For this review, take the finished solid that the model builds, in its own axes (mm). A direction names the side the tool comes from. Round coordinates to 2 decimals unless told otherwise and drop trailing zeros. Write each loop counter-clockwise with the first axis right and the second up, starting at its lowest first coordinate (ties: lowest second). Pieces come first, ordered by that corner, then holes. Notation, with made-up numbers: M -15,-6.5 L 40,-6.5 A26 cw 40,8.5 Z; hole C -36,77 d9. An arc over 180 degrees is marked long. Write each question's results on one line, items separated by ' | '. Start each with the question number.
Autodesk Inventor part; units mm, degrees
ref_plane "YZ Plane" through (0, 0, 0) normal (1, 0, 0) x (0, 1, 0)
ref_plane "XZ Plane" through (0, 0, 0) normal (0, 1, 0) x (-1, 0, 0)
ref_plane "XY Plane" through (0, 0, 0) normal (0, 0, 1) x (1, 0, 0)
sketch "Skizze1" plane through (0, 0, 0) normal (1, 0, 0) x (0, 1, 0)
  line L0 (0, -178.5) -> (0, 178.5)
  line L1 (-178.5, 0) -> (178.5, 0)
  line L2 (127.5, 127.5) -> (-127.5, 127.5)
  line L3 (-127.5, 127.5) -> (-127.5, -127.5)
  line L4 (-127.5, -127.5) -> (127.5, -127.5)
  line L5 (127.5, -127.5) -> (127.5, 127.5)
  point P0 (0, 0)
  dimension "d0" = 255
  dimension "d1" = 255
extrude "Extrusion1" add sketch "Skizze1" along normal mid plane 50
sketch "Skizze2" plane through (25, 0, 0) normal (1, 0, 0) x (0, 0, -1)
  line L0 (0, -178.5) -> (0, 178.5)
  line L1 (178.5, 0) -> (-178.5, 0)
  line L2 (-126, 126) -> (126, 126)
  line L3 (126, 126) -> (126, -126)
  line L4 (126, -126) -> (-126, -126)
  line L5 (-126, -126) -> (-126, 126)
  point P0 (0, 0)
  dimension "d4" = 252
  dimension "d5" = 252
extrude "Extrusion2" cut sketch "Skizze2" against normal blind 50
fillet "Rundung1" radius 2.5 4 edges at (0, 127.5, 127.5) (0, 127.5, -127.5) (0, -127.5, 127.5) (0, -127.5, -127.5)
fillet "Rundung2" radius 1 4 edges at (0, 126, 126) (0, 126, -126) (0, -126, -126) (0, -126, 126)
sketch "Skizze3" plane through (25, -126, 125) normal (0, 1, 0) x (1, 0, 0)
  circle A0 centre (-35, 51) radius 2
  circle A1 centre (-35, 199) radius 2
  line L0 (0, 0) -> (-50, 0)
  line L1 (-50, 0) -> (-50, 250)
  point P0 (-50, -1)
  dimension "d15" = 4
  dimension "d16" = 4
  dimension "d19" = 52
  dimension "d20" = 148
  dimension "d21" = 15
  dimension "d22" = 15
extrude "Extrusion3" add sketch "Skizze3" along normal blind 10
sketch "Skizze4" plane through (25, 126, -125) normal (0, -1, 0) x (1, 0, 0)
  circle A0 centre (-35, 51) radius 2
  circle A1 centre (-35, 199) radius 2
  line L0 (-50, 0) -> (-50, 250)
  point P0 (-25, 125)
  point P1 (-50, -1)
  dimension "d23" = 4
  dimension "d24" = 4
  dimension "d25" = 15
  dimension "d26" = 15
  dimension "d27" = 52
  dimension "d28" = 148
extrude "Extrusion4" add sketch "Skizze4" along normal blind 10
properties part number "Aussengehäuse" material "Stahl"
Item 1: Mouldability with a two-part tool opening along Z and no side actions: class faces 3 (the flat face through (0, -127.5, 2)), 4 (the flat face through (0, -2, 126)), 5 (the flat face through (0, -2, -127.5)) as pulls with the +Z half, pulls with the -Z half, needs draft (parallel to the pull), parting line crosses it, or undercut.
Item 2: For faces 1 (the flat face through (0, 127.5, -2)), 2 (the flat face through (0, 2, -126)), list the 3-axis set-ups (+Z, -Z, +X, -X, +Y, -Y) from which the entire face can be reached by the end or side of a thin tool; tool diameter is ignored.
Item 3: For probe 1 along Y at (x, z) = (19.5, -52), list the stretches that pass through material, from the lowest coordinate up.
Item 4: We need section A-A on z = -80.5. State the section outline as (x, y) points, then the cut area to 3 significant figures.
Item 5: We need section B-B on x = 18. State the section outline as (y, z) points, then the cut area to 3 significant figures.
Numbers:
1) face 3: needs draft | face 4: undercut | face 5: pulls with the -Z half
2) face 1: +Z, -Z, +X, -X, +Y | face 2: +X, -X
3) probe 1: y = -127.5 to -126, 126 to 127.5
4) outline: M -25,-127.5 L 25,-127.5 L 25,-126 L -25,-126 Z; M -25,126 L 25,126 L 25,127.5 L -25,127.5 Z | area: 150 mm^2
5) outline: M -127.5,-125 A2.5 ccw -125,-127.5 L 125,-127.5 A2.5 ccw 127.5,-125 L 127.5,125 A2.5 ccw 125,127.5 L -125,127.5 A2.5 ccw -127.5,125 Z; hole M -126,-125 A1 ccw -125,-126 L 125,-126 A1 ccw 126,-125 L 126,125 A1 ccw 125,126 L -125,126 A1 ccw -126,125 Z | area: 1,520 mm^2
